```python
from build123d import *

# Parameters (mm, degrees)
F0_R     = 10.55
F0_R_2   = 9.65
F1_DEPTH = 10
F3_DEPTH = 2.5


with BuildPart() as f1:
    # F0 (on Top) → F1 (new body)
    with BuildSketch(Plane.XY):
        Circle(F0_R)
        Circle(F0_R_2, mode=Mode.SUBTRACT)
    extrude(amount=F1_DEPTH)

    # F2 (on face) → F3 (join)
    with BuildSketch(Plane(origin=(0, 0, 0), x_dir=(1, 0, 0), z_dir=(0, 0, -1))):
        with BuildLine():
            ThreePointArc((-2.5, -8.124038), (-8.5, 0), (-2.5, 8.124038))
            Line((-2.5, 8.124038), (-2.5, 9.320542))
            ThreePointArc((-2.5, 9.320542), (-9.65, 0), (-2.5, -9.320542))
            Line((-2.5, -9.320542), (-2.5, -8.124038))
        make_face()
        with BuildLine():
            ThreePointArc((2.5, -9.320542), (9.65, 0), (2.5, 9.320542))
            Line((2.5, 9.320542), (2.5, 8.124038))
            ThreePointArc((2.5, 8.124038), (8.5, 0), (2.5, -8.124038))
            Line((2.5, -8.124038), (2.5, -9.320542))
        make_face()
    extrude(amount=-F3_DEPTH)


solid = f1.part
```
Read the model definition and answer for the solid it produces. Units are mm, in the model's axes. A direction names the side the tool comes from. Round coordinates to 2 decimals unless told otherwise and drop trailing zeros. Write each loop counter-clockwise with the first axis right and the second up, starting at its lowest first coordinate (ties: lowest second). Pieces come first, ordered by that corner, then holes. Notation, with made-up numbers: M -38.5,-22 L -24.5,-22 A15 ccw -24.5,-10 Z; hole C 37.25,83.25 d4. An arc over 180 degrees is marked long. One line per item, written item: value.
Q1. Find section A-A on x = 0. Write down the section's boundary in (y, z).
Data:
outline: M -10.55,0 L -9.65,0 L -9.65,10 L -10.55,10 Z; M 9.65,0 L 10.55,0 L 10.55,10 L 9.65,10 Z
Q2. Straight lines are drawn through the part: line 1 (Y direction, x = 0, z = 3.25); line 2 (Y direction, x = -7.5, z = 6); line 3 (X direction, y = -8, z = 5). For each, find the intervals that lie inside material, in ascending order. Write a range as [from, to].
Data:
line 1: [-10.55, -9.65], [9.65, 10.55]
line 2: [-7.42, -6.07], [6.07, 7.42]
line 3: [-6.88, -5.4], [5.4, 6.88]
Q3. Find section B-B on y = 0. Write down the section's boundary in (x, z).
Data:
outline: M -10.55,0 L -8.5,0 L -8.5,2.5 L -9.65,2.5 L -9.65,10 L -10.55,10 Z; M 8.5,0 L 10.55,0 L 10.55,10 L 9.65,10 L 9.65,2.5 L 8.5,2.5 Z
Q4. For a pull along X with two mould halves and no side action, classify faces 4 (the flat face through (5, -9, 10)), 5 (the cylindrical face through (10.063, 3.169, 4.93)), 6 (the flat face through (-9, -1, 2.5)) as +X half, -X half, draft (parallel to the pull), parting line (faces both ways), or undercut.
Data:
face 4: draft
face 5: parting line
face 6: undercut
Q5. Which of the six approach directions +Z, -Z, +X, -X, +Y, -Y give full straight-line access (tool end or side, diameter ignored) to faces 1 (the flat face through (2.5, 9, 1)), 2 (the flat face through (8, 4, 0)), 3 (the cylindrical face through (-9.64, 0.42, 6.04))?
Data:
face 1: +Z, -Z
face 2: -Z, +X, -X, +Y, -Y
face 3: +Z
Q6. Find section C-C on z = 1.25. Write down the section's boundary in (x, y).
Data:
outline: C 0,0 d21.1; hole M -2.5,-9.32 A9.65 ccw 2.5,-9.32 L 2.5,-8.12 A8.5 ccw 2.5,8.12 L 2.5,9.32 A9.65 ccw -2.5,9.32 L -2.5,8.12 A8.5 ccw -2.5,-8.12 Z
Q7. Flat-ended cylindrical pins translate along their axes: pin 1 Ø0.6 at (y, z) = (-9, 0.5) entering from -X; pin 2 Ø1 at (y, z) = (-9, 1.5) entering from +X; pin 3 Ø6 at (x, z) = (5, 7) entering from +Y. Find the tip coordinate at first contact, or state that the pin passes through.
Data:
pin 1: x = -5.97
pin 2: x = 6.25
pin 3: y = 10.36
Q8. Find section D-D on y = 3.5. Write down the section's boundary in (x, z), plus the area to 3 significant figures.
Data:
outline: M -9.95,0 L -7.75,0 L -7.75,2.5 L -8.99,2.5 L -8.99,10 L -9.95,10 Z; M 7.75,0 L 9.95,0 L 9.95,10 L 8.99,10 L 8.99,2.5 L 7.75,2.5 Z
area: 25.4 mm2
